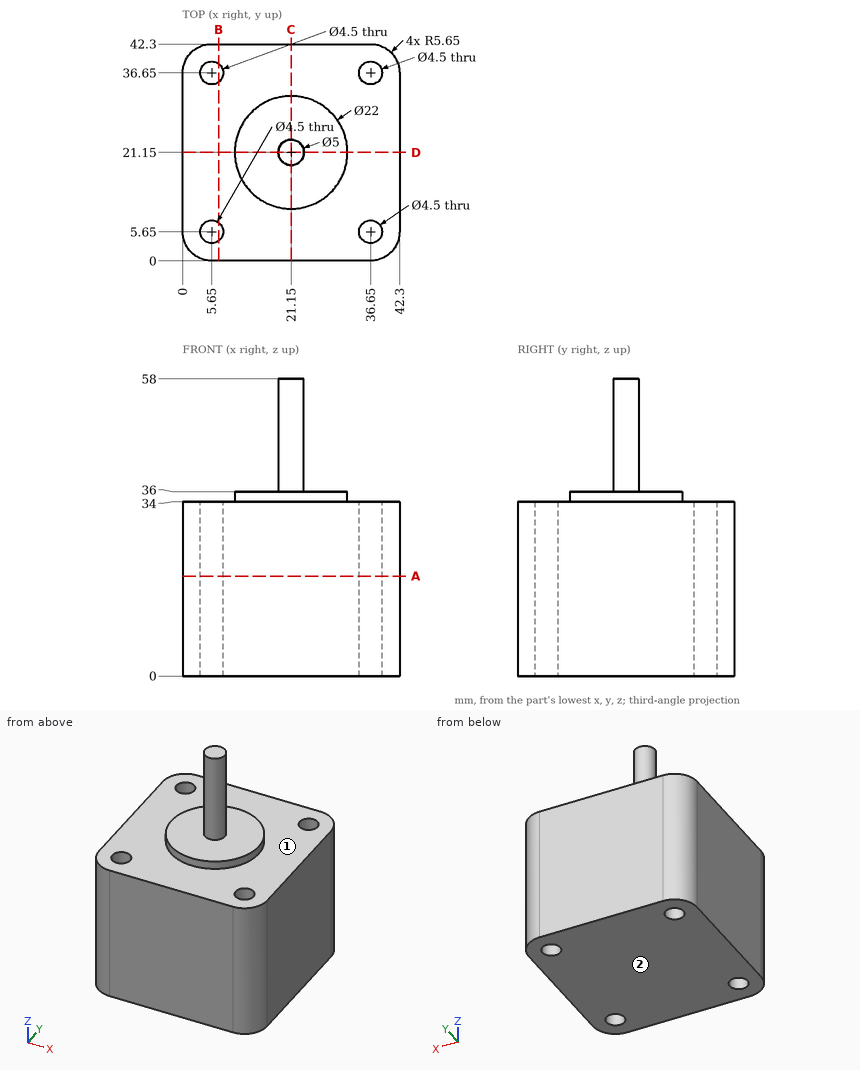
Input: dimensioned drawing with shaded views. Units: mm. Origin: part minimum x, y, z. A direction names the side the tool comes from. Coordinates: 2 decimals unless noted, no trailing zeros. Write each loop counter-clockwise with the first axis right and the second up, starting at its lowest first coordinate (ties: lowest second). Pieces come first, ordered by that corner, then holes. Notation, with made-up numbers: M 4.5,59.5 L 17.5,59.5 A7 ccw 17.5,63.5 Z; hole C 59,57.25 d8. An arc over 180 degrees is marked long. Use one line per item in the form item = value.
Q1. Section B-B (x = 7). Return loops of the section in (y, z).
Answer below:
outline = M 0,0 L 3.85,0 L 3.85,34 L 0,34 Z; M 7.45,0 L 34.85,0 L 34.85,34 L 7.45,34 Z; M 38.45,0 L 42.3,0 L 42.3,34 L 38.45,34 Z
Q2. Set-up query: the marked faces 1 and 2. Return all of +Z, -Z, +X, -X, +Y, -Y with unobstructed straight access to the full face (end or side cutting, diameter ignored); none if empty.
Answer below:
face_1 = +Z
face_2 = -Z, +X, -X, +Y, -Y
Q3. Section C-C (x = 21.15). Return loops of the section in (y, z), plus the area to 3 significant figures.
Answer below:
outline = M 0,0 L 42.3,0 L 42.3,34 L 32.15,34 L 32.15,36 L 23.65,36 L 23.65,58 L 18.65,58 L 18.65,36 L 10.15,36 L 10.15,34 L 0,34 Z
area = 1,590 mm²
Q4. Material intervals for probe 1 along Y at (x, z) = (36.65, 26); probe 2 along Y at (x, z) = (36, 26); probe 3 along X at (y, z) = (5, 33), sorted ascending. Write a range as from..to.
Answer below:
probe_1 = 0..3.4, 7.9..34.4, 38.9..42.3
probe_2 = 0..3.5, 7.8..34.5, 38.8..42.3
probe_3 = 0.04..3.5, 7.8..34.5, 38.8..42.26
Q5. First-contact query: pin 1 (4 mm diameter, centred on x = 17, z = 45.5, fed in from +Y); pin 2 (3 mm diameter, centred on x = 26, z = 50, fed in from +Y); pin 3 (1 mm diameter, centred on x = 7, y = 12, fed in from +Z). Flat tips, straight axial feed; report the tip coordinate or a pass-through.
Answer below:
pin_1 = 22.43
pin_2 = through
pin_3 = 34
Q6. Section A-A (z = 19.5). Return loops of the section in (x, y).
Answer below:
outline = M 0,5.65 A5.65 ccw 5.65,0 L 36.65,0 A5.65 ccw 42.3,5.65 L 42.3,36.65 A5.65 ccw 36.65,42.3 L 5.65,42.3 A5.65 ccw 0,36.65 Z; hole C 5.65,5.65 d4.5; hole C 5.65,36.65 d4.5; hole C 36.65,5.65 d4.5; hole C 36.65,36.65 d4.5
